from build123d import *

# Parameters (mm, degrees)
CROQUIS1_R              = 9
SALIENTE_EXTRUIR1_DEPTH = 17
CROQUIS2_R              = 6
SALIENTE_EXTRUIR2_DEPTH = 9
CORTAR_EXTRUIR1_DEPTH   = 9.5
CROQUIS4_R              = 2.25
SALIENTE_EXTRUIR3_DEPTH = 7
CROQUIS5_R              = 1.65
SALIENTE_EXTRUIR4_DEPTH = 4
CROQUIS6_R              = 2.05
CORTAR_EXTRUIR2_DEPTH   = 5


with BuildPart() as part:
    # Croquis1 → Saliente-Extruir1 (new body)
    with BuildSketch(Plane(origin=(0, 0, 0), x_dir=(1, 0, 0), z_dir=(0, 1, 0))):
        with Locations(Location((0, 0, 0), (0, 0, 270))):
            Circle(CROQUIS1_R)
    extrude(amount=SALIENTE_EXTRUIR1_DEPTH)

    # Croquis2 → Saliente-Extruir2 (add)
    with BuildSketch(Plane(origin=(0, 17, 0), x_dir=(1, 0, 0), z_dir=(0, 1, 0))):
        with Locations(Location((0, 0, 0), (0, 0, 270))):
            Circle(CROQUIS2_R)
    extrude(amount=SALIENTE_EXTRUIR2_DEPTH)

    # Croquis3 → Cortar-Extruir1 (cut, symmetric)
    with BuildSketch(Plane.XY):
        Polygon((-6, 24.801), (0, 25.6), (6, 26), (-6, 26), align=None)
    extrude(amount=CORTAR_EXTRUIR1_DEPTH, both=True, mode=Mode.SUBTRACT)

    # Croquis4 → Saliente-Extruir3 (add)
    with BuildSketch(Plane(origin=(-1.699115044, 25.486725664, 0), x_dir=(0.997785157856609, 0.06651901052377411, 0), z_dir=(-0.06651901052377411, 0.997785157856609, 0))):
        with Locations(Location((0.629712535, 2.694122729, 0), (0, 0, 298.487451849))):
            Circle(CROQUIS4_R)
        with Locations(Location((0.970047848, -2.805877271, 0), (0, 0, 70.99163809))):
            Circle(CROQUIS4_R)
    extrude(amount=SALIENTE_EXTRUIR3_DEPTH)

    # Croquis5 → Saliente-Extruir4 (add)
    with BuildSketch(Plane(origin=(-2.164748118, 32.471221769, 0), x_dir=(0.997785157856609, 0.06651901052377412, 0), z_dir=(-0.06651901052377412, 0.997785157856609, 0))):
        with Locations(Location((0.629712535, 2.694122729, 0), (0, 0, 180))):
            Circle(CROQUIS5_R)
        with Locations(Location((0.970047848, -2.805877271, 0), (0, 0, 180))):
            Circle(CROQUIS5_R)
    extrude(amount=SALIENTE_EXTRUIR4_DEPTH)

    # Croquis6 → Cortar-Extruir2 (cut)
    with BuildSketch(Plane.XZ):
        with Locations(Location((0, 0, 0), (0, 0, 270))):
            Circle(CROQUIS6_R)
    extrude(amount=-CORTAR_EXTRUIR2_DEPTH, mode=Mode.SUBTRACT)


solid = part.part
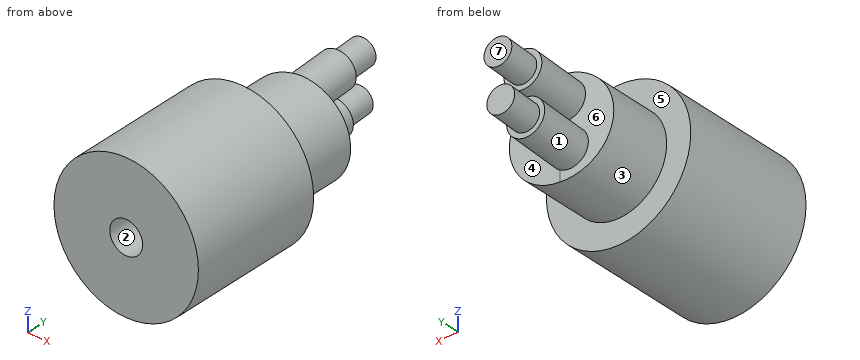
Geometry: final body of the model. Coordinates: model frame, mm. Face numbers are marked on the shaded views. A direction names the side the tool comes from. Round coordinates to 2 decimals unless told otherwise and drop trailing zeros. Loops run counter-clockwise (first coordinate to the right, second up) from the corner with the lowest first, then second, coordinate; pieces in that order, holes last. Notation, with made-up numbers: M 21.25,70 L 66.25,70 A24 cw 66.25,95 Z; hole C -22,46 d3. An arc over 180 degrees is marked long. Put each result on its own line as item: value. Start each with the question number.
(1) Set-up query: the marked faces 1, 2 and 3. Return all of +Z, -Z, +X, -X, +Y, -Y with unobstructed straight access to the full face (end or side cutting, diameter ignored); none if empty.
(2) Draft query along X for the marked faces 4, 5, 6 and 7. Return one class per face: +X half, -X half, draft (parallel to the pull), parting line (faces both ways), or undercut.
(3) Section query D-D (x = -7.5). Return loops of the section in (y, z), then the cut area to 3 significant figures.
(4) Section query A-A (z = 0). Return loops of the section in (x, y), then the cut area to 3 significant figures.
(5) Material intervals for line 1 along X through (y, z) = (1.55, 0); line 2 along Y through (x, z) = (-4.5, 7.25); line 3 along X through (y, z) = (2.5, -1.25), sorted ascending. Write a range as [from, to].
(6) Contact query for flat-ended pins moving along their axis: pin 1 Ø6 at (y, z) = (32, 0) entering from +X; pin 2 Ø3 at (x, y) = (-4.5, 8.5) entering from -Z; pin 3 Ø1.5 at (x, y) = (1, 4.5) entering from +Z. Output: stop coordinate, or through.
(7) Section query B-B (y = 3.5). Return loops of the section in (x, z), then the cut area to 3 significant figures.
(8) Section query C-C (y = 14.5). Return loops of the section in (x, z).
Findings below:
1. face 1: none
1. face 2: -Y
1. face 3: +Y
2. face 4: undercut
2. face 5: draft
2. face 6: undercut
2. face 7: -X half
3. outline: M 0,-4.97 L 17,-4.97 L 17,4.97 L 0,4.97 Z
3. area: 169 mm2
4. outline: M -9,0 L -2.05,0 L -2.05,5 L 2.05,5 L 2.05,0 L 9,0 L 9,17 L 6,17 L 6,26 L 0,25.6 L -6,24.8 L -6,17 L -9,17 Z
4. area: 388 mm2
5. line 1: x = [-9, -2.05], [2.05, 9]
5. line 2: y = [0, 17]
5. line 3: x = [-8.91, -1.62], [1.62, 8.91]
6. pin 1: stops at x = 1.18
6. pin 2: stops at z = -8.49
6. pin 3: stops at z = 9
7. outline: C 0,0 d18; hole C 0,0 d4.1
7. area: 241 mm2
8. outline: C 0,0 d18
